```python
from build123d import *

# Parameters (mm, degrees)
F1_DEPTH = 10
F2_R     = 3.25
F3_DEPTH = 25
F5_DEPTH = 3
F7_DEPTH = 3


with BuildPart() as f1:
    # F0 (on Front) → F1 (new body, symmetric)
    with BuildSketch(Plane.XZ):
        with BuildLine():
            Line((0, 3), (0, 0))
            Line((0, 0), (20.171573, 0))
            ThreePointArc((20.171573, 0), (22.019332, 1.234633), (21.585786, 3.414214))
            Line((21.585786, 3.414214), (10.857864, 14.142136))
            Line((10.857864, 14.142136), (3.786797, 7.071068))
            Line((3.786797, 7.071068), (4.443651, 6.414214))
            ThreePointArc((4.443651, 6.414214), (4.877196, 4.234633), (3.029437, 3))
            Line((3.029437, 3), (0, 3))
        make_face()
    extrude(amount=F1_DEPTH, both=True)

    # F2 (on face) → F3 (cut)
    with BuildSketch(Plane(origin=(-1.642136, 0, 1.642136), x_dir=(0, -1, 0), z_dir=(-0.707107, 0, 0.707107))):
        with Locations((-4, 12.67767)):
            Circle(F2_R)
        with Locations((4, 12.67767)):
            Circle(F2_R)
    extrude(amount=-F3_DEPTH, mode=Mode.SUBTRACT)

    # F4 (on Top) → F5 (join)
    with BuildSketch(Plane.XY):
        with BuildLine():
            Line((0, -10), (0, 10))
            Line((0, 10), (-16.533815, 10))
            ThreePointArc((-16.533815, 10), (-35, 21), (-53.466185, 10))
            Line((-53.466185, 10), (-68, 10))
            ThreePointArc((-68, 10), (-69.414214, 9.414214), (-70, 8))
            Line((-70, 8), (-70, -8))
            ThreePointArc((-70, -8), (-69.414214, -9.414214), (-68, -10))
            Line((-68, -10), (-53.466185, -10))
            ThreePointArc((-53.466185, -10), (-35, -21), (-16.533815, -10))
            Line((-16.533815, -10), (0, -10))
        make_face()
        with BuildLine():
            ThreePointArc((-21.562904, -6.666667), (-35, -15), (-48.437096, -6.666667))
            ThreePointArc((-48.437096, -6.666667), (-49.543377, -5.45049), (-51.124515, -5))
            Line((-51.124515, -5), (-62, -5))
            ThreePointArc((-62, -5), (-64.12132, -4.12132), (-65, -2))
            Line((-65, -2), (-65, 2))
            ThreePointArc((-65, 2), (-64.12132, 4.12132), (-62, 5))
            Line((-62, 5), (-51.124515, 5))
            ThreePointArc((-51.124515, 5), (-49.543377, 5.45049), (-48.437096, 6.666667))
            ThreePointArc((-48.437096, 6.666667), (-35, 15), (-21.562904, 6.666667))
            ThreePointArc((-21.562904, 6.666667), (-20.456623, 5.45049), (-18.875485, 5))
            Line((-18.875485, 5), (-8, 5))
            ThreePointArc((-8, 5), (-5.87868, 4.12132), (-5, 2))
            Line((-5, 2), (-5, -2))
            ThreePointArc((-5, -2), (-5.87868, -4.12132), (-8, -5))
            Line((-8, -5), (-18.875485, -5))
            ThreePointArc((-18.875485, -5), (-20.456623, -5.45049), (-21.562904, -6.666667))
        make_face(mode=Mode.SUBTRACT)
    extrude(amount=F5_DEPTH)

    # F6 (on face) → F7 (join)
    with BuildSketch(Plane.XY.offset(3)):
        with BuildLine():
            ThreePointArc((-51.707501, 9.047619), (-35, 19), (-18.292499, 9.047619))
            Line((-18.292499, 9.047619), (-16.533815, 10))
            ThreePointArc((-16.533815, 10), (-35, 21), (-53.466185, 10))
            Line((-53.466185, 10), (-51.707501, 9.047619))
        make_face()
        with BuildLine():
            Line((-16.533815, -10), (-18.292499, -9.047619))
            ThreePointArc((-18.292499, -9.047619), (-35, -19), (-51.707501, -9.047619))
            Line((-51.707501, -9.047619), (-53.466185, -10))
            ThreePointArc((-53.466185, -10), (-35, -21), (-16.533815, -10))
        make_face()
    extrude(amount=F7_DEPTH)


solid = f1.part
```
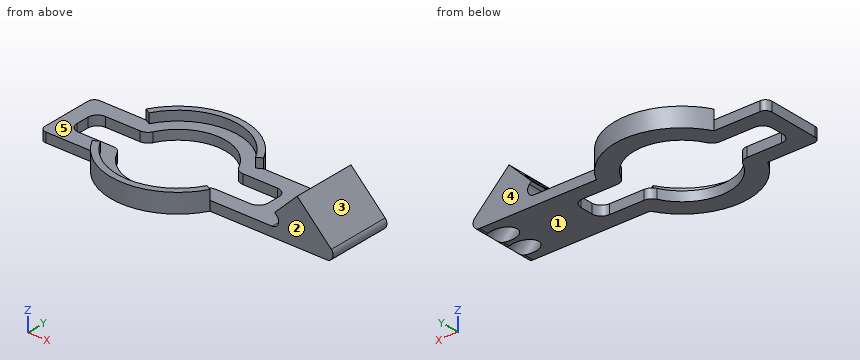
Part model, mm, in its own coordinate system. Face numbers are marked on the shaded views. A direction names the side the tool comes from. Round coordinates to 2 decimals unless told otherwise and drop trailing zeros. Loops run counter-clockwise (first coordinate to the right, second up) from the corner with the lowest first, then second, coordinate; pieces in that order, holes last. Notation, with made-up numbers: (85.5, 20.25) -> (98.5, 20.25) arc R25 ccw to (98.5, 34.25) -> close; hole circle Ø6 at (6.5, 88). An arc over 180 degrees is marked (long way). Use one line per item in the form item = value. Start each with the question number.
Item 1: Drop flat-ended pins along their axis: pin 1 Ø8 at (x, y) = (-51, 12) entering from +Z; pin 2 Ø3.5 at (x, z) = (-15.5, 1) entering from -Y; pin 3 Ø2.5 at (x, z) = (-58.5, 2) entering from +Y. Give the stop position or say it passes through.
Item 2: Band-saw the part on D-D (x = -36.5). List the corners of the cut face in (y, z).
Item 3: Band-saw the part on C-C (y = 3). List the corners of the cut face in (x, z).
Item 4: Band-saw the part on B-B (y = -13.5). List the corners of the cut face in (x, z), plus the area to 3 significant figures.
Item 5: Tool access for the marked faces 1 and 2: list every direction of +Z, -Z, +X, -X, +Y, -Y with a clear straight run to the whole face (end or side of a thin tool).
Item 6: Drill centre lines: line 1 along Y through (x, z) = (-34.5, 5); line 2 along Y through (x, z) = (-12, 1.5); line 3 along X through (y, z) = (5.5, 1). Where is each one in solid material? Low to high.
Item 7: Two-plate mould, pull along Y, no slides. Class the marked faces 3, 4 and 5: released by +Y, released by -Y, zero draft, split by the parting line, or undercut.
Item 8: Band-saw the part on A-A (x = -58.5). List the corners of the cut face in (y, z), plus the area to 3 significant figures.
Data:
q1.pin_1 = 6
q1.pin_2 = -11.22
q1.pin_3 = 10
q2.outline = (-20.95, 0) -> (-14.92, 0) -> (-14.92, 3) -> (-18.94, 3) -> (-18.94, 6) -> (-20.95, 6) -> close; (14.92, 0) -> (20.95, 0) -> (20.95, 6) -> (18.94, 6) -> (18.94, 3) -> (14.92, 3) -> close
q3.outline = (-70, 0) -> (-64.83, 0) -> (-64.83, 3) -> (-70, 3) -> close; (-5.17, 0) -> (13.56, 0) -> (5.14, 8.42) -> (3.79, 7.07) -> (4.44, 6.41) arc R2 cw to (3.03, 3) -> (-5.17, 3) -> close; (9.51, 12.79) -> (21.65, 0.65) arc R2 ccw to (21.59, 3.41) -> (10.86, 14.14) -> close
q4.outline = (-51.09, 0) -> (-41.54, 0) -> (-41.54, 3) -> (-48.37, 3) -> (-48.37, 6) -> (-51.09, 6) -> close; (-28.46, 0) -> (-18.91, 0) -> (-18.91, 6) -> (-21.63, 6) -> (-21.63, 3) -> (-28.46, 3) -> close
q4.area = 73.6 mm^2
q5.face_1 = -Z, +X, -X, +Y, -Y
q5.face_2 = +Z, -Z, +X, -Y
q6.line_1 = -20.99 to -18.99, 18.99 to 20.99
q6.line_2 = -10 to -5, 5 to 10
q6.line_3 = -70 to -49.47, -20.53 to 12.85, 21.01 to 21.9
q7.face_3 = zero draft
q7.face_4 = released by +Y
q7.face_5 = undercut
q8.outline = (-10, 0) -> (-5, 0) -> (-5, 3) -> (-10, 3) -> close; (5, 0) -> (10, 0) -> (10, 3) -> (5, 3) -> close
q8.area = 30.0 mm^2
